Job drawing, mm, ordinate dimensions from the low corner. One solid piece. Give positions to 0.01 mm unless a question says otherwise; leave off trailing zeros. Order: outer loops, then holes, each group sorted by start corner. A loop starts at its lowest first (then second) coordinate and runs counter-clockwise, first axis right, second up. Notation, with made-up numbers: (88, 55) - (129, 55) arc R24 cw to (129, 68) - close; hole circle Ø6 at (84.5, -19). An arc over 180 degrees is marked (long way). Write each question's results on one line, items separated by ' | '. Start each with the question number.
1) Cut at A-A on y = 1.5. List the corners of the cut face in (x, z).
2) Cut at B-B on z = 41.5. List the corners of the cut face in (x, y).
3) Two-plate mould, pull along X, no slides. Class the marked faces 1 and 2: +X half, -X half, draft (parallel to the pull), parting line (faces both ways), or undercut.
4) Drop a flat-ended pin along its axis: pin 1 Ø10 at (x, z) = (8.5, 16.5) entering from -Y. Give the stop position or say it passes through.
5) Cut at C-C on x = 10.5. List the corners of the cut face in (y, z).
6) Drill centre lines: line 1 along Z through (x, y) = (7.5, 2.5); line 2 along X through (y, z) = (2, 24); line 3 along Y through (x, z) = (13.25, 39). Where is each one in solid material? Low to high. Write a range as from..to.
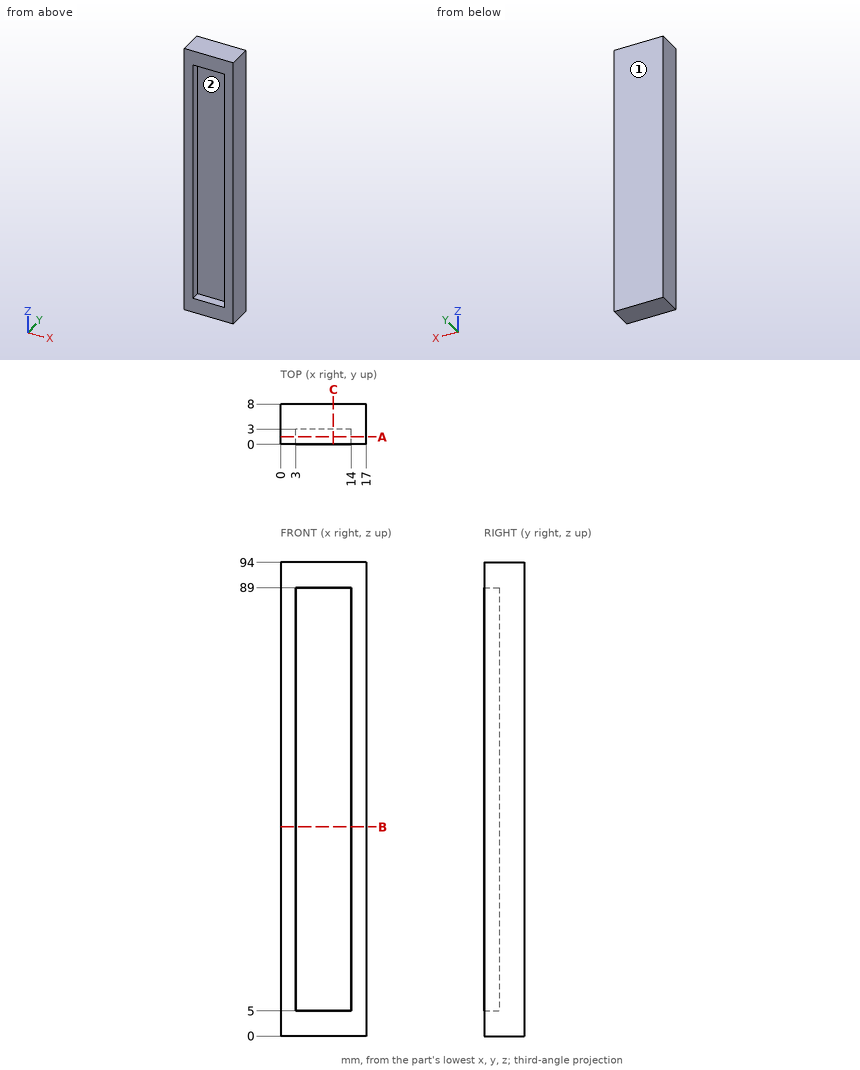
Results:
1) outline: (0, 0) - (17, 0) - (17, 94) - (0, 94) - close; hole (3, 5) - (14, 5) - (14, 89) - (3, 89) - close
2) outline: (0, 0) - (3, 0) - (3, 3) - (14, 3) - (14, 0) - (17, 0) - (17, 8) - (0, 8) - close
3) face 1: draft | face 2: undercut
4) pin 1: y = 3
5) outline: (0, 0) - (8, 0) - (8, 94) - (0, 94) - (0, 89) - (3, 89) - (3, 5) - (0, 5) - close
6) line 1: 0..5, 89..94 | line 2: 0..3, 14..17 | line 3: 3..8
